```python
from build123d import *

# Parameters (mm, degrees)
BOSS_EXTRUDE2_DEPTH = 5.4
BOSS_EXTRUDE3_DEPTH = 5.4


with BuildPart() as part:
    # Sketch1 → Boss-Extrude2 (new body)
    with BuildSketch(Plane(origin=(0, 0, 0), x_dir=(0, 0, -1), z_dir=(1, 0, 0))):
        Polygon((142.9875, 130), (-7.0375, 130), (-7.0375, 9.3375), (-12.4375, 9.3375), (-12.4375, 130), (-148.3875, 130), (-148.3875, 81.735), (-153.7875, 81.735), (-153.7875, 33.47), (-148.3875, 33.47), (-148.3875, -14.795), (-153.7875, -14.795), (-153.7875, -63.06), (-148.3875, -63.06), (-148.3875, -111.325), (142.9875, -111.325), (142.9875, -63.06), (148.3875, -63.06), (148.3875, -14.795), (142.9875, -14.795), (142.9875, 33.47), (148.3875, 33.47), (148.3875, 81.735), (142.9875, 81.735), align=None)
    extrude(amount=BOSS_EXTRUDE2_DEPTH)

    # Sketch2 → Boss-Extrude3 (add)
    with BuildSketch(Plane(origin=(5.4, 0, 0), x_dir=(0, 0, -1), z_dir=(1, 0, 0))):
        Polygon((-148.42814, -111.36564), (143.02814, -111.36564), (143.02814, -63.10064), (148.42814, -63.10064), (148.42814, -14.75436), (143.02814, -14.75436), (143.02814, 33.42936), (148.42814, 33.42936), (148.42814, 81.77564), (143.02814, 81.77564), (143.02814, 130.04064), (-7.07814, 130.04064), (-7.07814, 9.37814), (-12.39686, 9.37814), (-12.39686, 130.04064), (-148.42814, 130.04064), (-148.42814, 81.77564), (-153.82814, 81.77564), (-153.82814, 33.42936), (-148.42814, 33.42936), (-148.42814, -14.75436), (-153.82814, -14.75436), (-153.82814, -63.10064), (-148.42814, -63.10064), align=None)
    extrude(amount=-BOSS_EXTRUDE3_DEPTH)


solid = part.part
```
Design review of the part built by this model. Coordinates are the model's own, in mm. Give positions to 0.01 mm unless a question says otherwise; leave off trailing zeros. Loops run counter-clockwise (first coordinate to the right, second up) from the corner with the lowest first, then second, coordinate; pieces in that order, holes last. Notation, with made-up numbers: M -35,14 L 20,14 A19 ccw 20,37 Z; hole C 46.5,-30 d10. An arc over 180 degrees is marked long. Return JSON: item names as keys, results as strings. Group by question number.
Item 1: We need section C-C (y = -89). Give the boundary of the cut face in (x, z).
Item 2: For probe 1 along Z at (x, y) = (0.35, 79.5); probe 2 along Z at (x, y) = (2.9, 104.5); probe 3 along Z at (x, y) = (0.7, -67), list the stretches that pass through material, from the lowest coordinate up.
Item 3: Insertion check: pin 1 Ø1.6 at (x, y) = (4, 109.5) entering from -Z; pin 2 Ø1.6 at (x, y) = (3, 3.5) entering from +Z; pin 3 Ø2.5 at (x, z) = (3, 150.5) entering from -Y. Each pin has a flat end and moves straight along its axis. Give the tip position at first contact, or say it passes through.
Item 4: We need section A-A (y = 61). Give the boundary of the cut face in (x, z), and give its area (3 significant figures).
Item 5: We need section B-B (x = 1.8). Give the boundary of the cut face in (y, z).
Output:
{
 "1": {"outline": "M 0,-143.03 L 5.4,-143.03 L 5.4,148.43 L 0,148.43 Z"},
 "2": {"probe 1": "z = -148.43 to 7.08, 12.4 to 153.83", "probe 2": "z = -143.03 to 7.08, 12.4 to 148.43", "probe 3": "z = -143.03 to 148.43"},
 "3": {"pin 1": "stops at z = -143.03", "pin 2": "stops at z = 148.43", "pin 3": "stops at y = -63.1"},
 "4": {"outline": "M 0,-148.43 L 5.4,-148.43 L 5.4,7.08 L 0,7.08 Z; M 0,12.4 L 5.4,12.4 L 5.4,153.83 L 0,153.83 Z", "area": "1,600 mm^2"},
 "5": {"outline": "M -111.37,-143.03 L -63.1,-143.03 L -63.1,-148.43 L -14.75,-148.43 L -14.75,-143.03 L 33.43,-143.03 L 33.43,-148.43 L 81.78,-148.43 L 81.78,-143.03 L 130.04,-143.03 L 130.04,7.08 L 9.38,7.08 L 9.38,12.4 L 130.04,12.4 L 130.04,148.43 L 81.78,148.43 L 81.78,153.83 L 33.43,153.83 L 33.43,148.43 L -14.75,148.43 L -14.75,153.83 L -63.1,153.83 L -63.1,148.43 L -111.37,148.43 Z"}
}
